Could you check a few things on this model? Use its own coordinates, in mm. A direction names the side the tool comes from. Give positions to 0.01 mm unless a question says otherwise; leave off trailing zeros. Order: outer loops, then holes, each group sorted by start corner. A loop starts at its lowest first (then second) coordinate and runs counter-clockwise, first axis right, second up. Notation, with made-up numbers: (14, -13.75) - (47, -13.75) arc R26 cw to (47, 10.25) - close; hole circle Ø11 at (-39.75, 15). An arc over 180 degrees is marked (long way). One line per question, with ' | ' between items. Start each with the question number.
1. Imagine slicing it at D-D (x = 16). Please give me the cut outline in (y, z).
2. If we mould it in two halves opening along Y, with no side actions, what happens to faces 1 (the flat face through (-17, -22, -13)), 2 (the cylindrical face through (-18, -9, 14)), 3 (the flat face through (5, -45, 7))? For each: released by +Y, released by -Y, zero draft, split by the parting line, or undercut.
3. I need wall thicknesses on probe 1 along Y at (x, z) = (-16, 14.75); probe 2 along X at (y, z) = (-9, -9); probe 3 along X at (y, z) = (-37, 13). Which ranges of each line are inside material? Lowest first, please. Write a range as from..to.
4. Imagine slicing it at A-A (z = 11). Please give me the cut outline in (x, y), and give its area (3 significant figures).
5. Which directions (+Z, -Z, +X, -X, +Y, -Y) give clear straight access to the entire face, cutting with the end or side of a thin tool? Please do faces 4 (the flat face through (17, -22, -13)), 5 (the flat face through (7.794, -22.185, -9.575)), 6 (the cylindrical face through (13.5, -7.4, 14.1)).
6. Imagine slicing it at C-C (z = -3.5). Please give me the cut outline in (x, y), and give its area (3 significant figures).
7. Imagine slicing it at B-B (y = -24). Please give me the cut outline in (x, z) (3 decimals), and give its area (3 significant figures).
8. For P1, Ø2.5, axis at x = 16, y = -7.5, coming from the +Z side; P2, Ø1.5, axis at x = -3.5, z = -6, coming from the +Y side, each with a flat end and sliding along its axis, tell me the tip position at first contact or that it passes through.
```python
from build123d import *

# Parameters (mm, degrees)
F1_DEPTH = 45
F2_R     = 2.5
F3_DEPTH = 12


with BuildPart() as f1:
    # F0 (on Front) → F1 (new body)
    with BuildSketch(Plane.XZ):
        with BuildLine():
            Line((0, 20), (-22.5, 20))
            Line((-22.5, 20), (-22.5, -13))
            Line((-22.5, -13), (-10.66812, -13))
            Line((-10.66812, -13), (-5, -6.244998))
            ThreePointArc((-5, -6.244998), (-7.548509, 2.64953), (0, 8))
            Line((0, 8), (0, 20))
        make_face()
        with BuildLine():
            Line((22.5, 20), (0, 20))
            Line((0, 20), (0, 8))
            ThreePointArc((0, 8), (7.548509, 2.64953), (5, -6.244998))
            Line((5, -6.244998), (10.66812, -13))
            Line((10.66812, -13), (22.5, -13))
            Line((22.5, -13), (22.5, 20))
        make_face()
    extrude(amount=F1_DEPTH)

    # F2 (on face) → F3 (cut)
    with BuildSketch(Plane.XY.offset(20)):
        with Locations((-16, -7.5)):
            Circle(F2_R)
        with Locations((16, -7.5)):
            Circle(F2_R)
        with Locations((16, -37.5)):
            Circle(F2_R)
        with Locations((-16, -37.5)):
            Circle(F2_R)
    extrude(amount=-F3_DEPTH, mode=Mode.SUBTRACT)


solid = f1.part
```
Results found:
1) outline: (-45, -13) - (0, -13) - (0, 20) - (-5, 20) - (-5, 8) - (-10, 8) - (-10, 20) - (-35, 20) - (-35, 8) - (-40, 8) - (-40, 20) - (-45, 20) - close
2) face 1: zero draft | face 2: undercut | face 3: released by -Y
3) probe 1: y = -45..-40, -35..-10, -5..0 | probe 2: x = -22.5..-7.31, 7.31..22.5 | probe 3: x = -22.5..-18.45, -13.55..13.55, 18.45..22.5
4) outline: (-22.5, -45) - (22.5, -45) - (22.5, 0) - (-22.5, 0) - close; hole circle Ø5 at (-16, -37.5); hole circle Ø5 at (-16, -7.5); hole circle Ø5 at (16, -37.5); hole circle Ø5 at (16, -7.5) | area: 1,950 mm2
5) face 4: -Z, +X, -X, +Y, -Y | face 5: -Z, +Y, -Y | face 6: +Z
6) outline: (-22.5, -45) - (-7.19, -45) - (-7.19, 0) - (-22.5, 0) - close; (7.19, -45) - (22.5, -45) - (22.5, 0) - (7.19, 0) - close | area: 1,380 mm2
7) outline: (-22.5, -13) - (-10.668, -13) - (-5, -6.245) arc R8 cw (long way) to (5, -6.245) - (10.668, -13) - (22.5, -13) - (22.5, 20) - (-22.5, 20) - close | area: 1,190 mm2
8) P1: stops at z = 8 | P2: passes through
